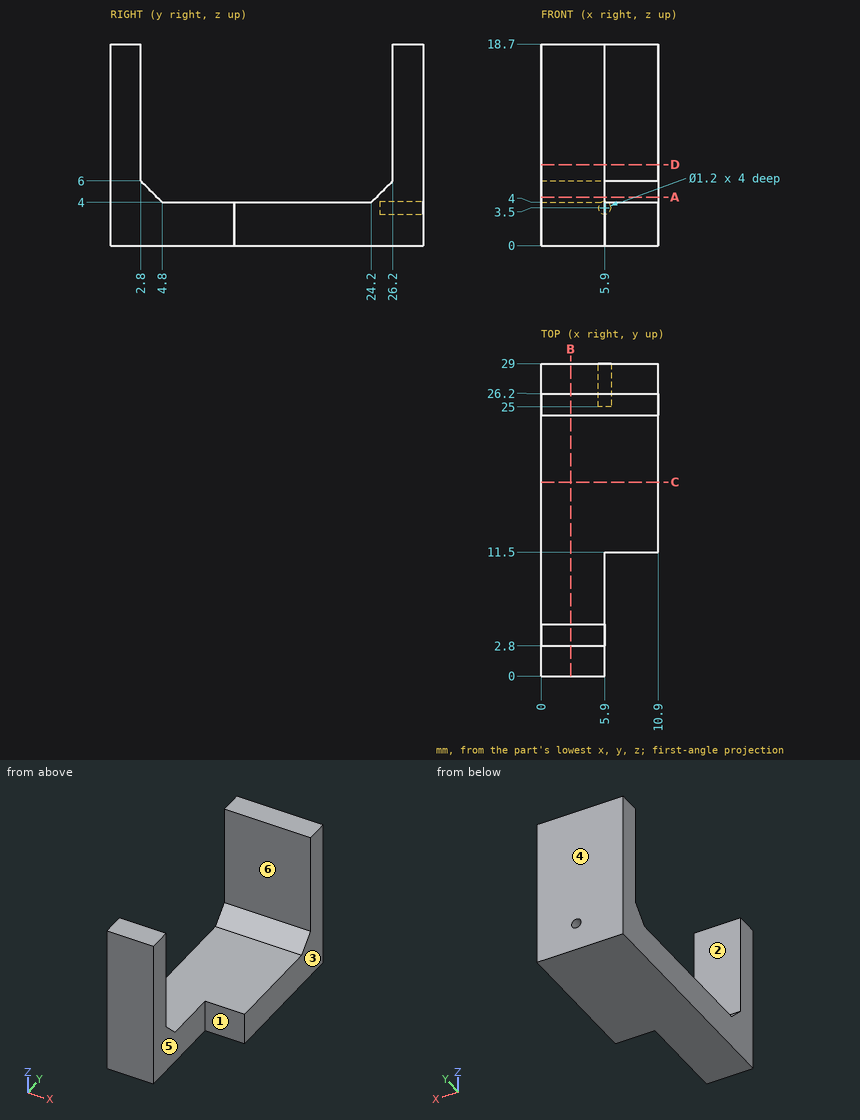
Design review of the part shown in the three views and the two pictorial views. Dimensions are in mm from the part's minimum x, y and z. A direction names the side the tool comes from. Round coordinates to 2 decimals unless told otherwise and drop trailing zeros. Order: outer loops, then holes, each group sorted by start corner. A loop starts at its lowest first (then second) coordinate and runs counter-clockwise, first axis right, second up. Notation, with made-up numbers: (78.25, 24) -> (83.25, 24) arc R26 ccw to (83.25, 53) -> close; hole circle Ø4 at (34.25, 57.5). An arc over 180 degrees is marked (long way). Write item = value, one per line. Start each with the question number.
1) Take a section at D-D on z = 7.5. State the section outline as (x, y) points.
2) Tool access review of the marked faces 4, 5 and 6: name each direction out of +Z, -Z, +X, -X, +Y, -Y from which nothing blocks a thin tool from reaching the whole face with its end or side.
3) Take a section at A-A on z = 4.5. State the section outline as (x, y) points, plus the area to 3 significant figures.
4) Take a section at B-B on x = 2.75. State the section outline as (y, z) points.
5) The part is to be moulded in two halves that separate along Y. For the marked faces 1, 2 and 3, say which applies: +Y half, -Y half, draft (parallel to the pull), parting line (faces both ways), or undercut.
6) To check wall thickness, follow line 1 (Z direction, x = 5.9, y = 26.9); line 2 (Y direction, x = 1.25, z = 12); line 3 (Z direction, x = 5.9, y = 26.1). State the ranges of each line that lie inside material, in increasing order. Write a range as from..to.
7) Insertion check: pin 1 (3 mm diameter, centred on x = 9.5, z = 2, fed in from -Y); pin 2 (0.7 mm diameter, centred on x = 5.9, z = 3.5, fed in from +Y); pin 3 (9 mm diameter, centred on y = 7, z = 10.5, fed in from +X). Each pin has a flat end and moves straight along its axis. Give the tip position at first contact, or say it passes through.
8) Take a section at C-C on y = 18. State the section outline as (x, z) points, plus the area to 3 significant figures.
Verdict:
q1.outline = (0, 0) -> (5.9, 0) -> (5.9, 2.8) -> (0, 2.8) -> close; (0, 26.2) -> (10.9, 26.2) -> (10.9, 29) -> (0, 29) -> close
q2.face_4 = +Z, -Z, +X, -X, +Y
q2.face_5 = +Z, -Z, +X, -Y
q2.face_6 = +Z, +X, -X
q3.outline = (0, 0) -> (5.9, 0) -> (5.9, 4.3) -> (0, 4.3) -> close; (0, 24.7) -> (10.9, 24.7) -> (10.9, 29) -> (0, 29) -> close
q3.area = 72.2 mm2
q4.outline = (0, 0) -> (29, 0) -> (29, 18.7) -> (26.2, 18.7) -> (26.2, 6) -> (24.2, 4) -> (4.8, 4) -> (2.8, 6) -> (2.8, 18.7) -> (0, 18.7) -> close
q5.face_1 = -Y half
q5.face_2 = undercut
q5.face_3 = draft
q6.line_1 = 0..2.9, 4.1..18.7
q6.line_2 = 0..2.8, 26.2..29
q6.line_3 = 0..2.9, 4.1..5.9
q7.pin_1 = 11.5
q7.pin_2 = 25
q7.pin_3 = 5.9
q8.outline = (0, 0) -> (10.9, 0) -> (10.9, 4) -> (0, 4) -> close
q8.area = 43.6 mm2
